Autodesk Inventor part; units mm, degrees
ref_plane "YZ Plane" through (0, 0, 0) normal (1, 0, 0) x (0, 1, 0)
ref_plane "XZ Plane" through (0, 0, 0) normal (0, 1, 0) x (-1, 0, 0)
ref_plane "XY Plane" through (0, 0, 0) normal (0, 0, 1) x (1, 0, 0)
sketch "スケッチ1" plane through (0, 0, 0) normal (0, 0, 1) x (1, 0, 0)
  line L0 (0, 2.3094) -> (2, 1.1547)
  line L1 (2, 1.1547) -> (2, -1.1547)
  line L2 (2, -1.1547) -> (0, -2.3094)
  line L3 (0, -2.3094) -> (-2, -1.1547)
  line L4 (-2, -1.1547) -> (-2, 1.1547)
  line L5 (-2, 1.1547) -> (0, 2.3094)
  point P0 (0, 0)
  point P1 (0, 0)
  dimension "d0" = 4
extrude "押し出し1" add sketch "スケッチ1" along normal blind 6
sketch "スケッチ2" plane through (0, 0, 6) normal (0, 0, 1) x (1, 0, 0)
  circle A0 centre (0, 0) radius 1
  dimension "d3" = 2
extrude "押し出し2" add sketch "スケッチ2" along normal blind 5
thread "ねじ1"
sketch "スケッチ3" plane through (0, 0, 0) normal (0, 0, -1) x (-1, 0, 0)
  point P0 (0, 0)
hole "穴1" at (0, 0, 0) direction (0, 0, 1) diameter 1.567 depth 4 tip angle 118
properties part number "ジュラコンスペーサー（六角）_BS-2006E" material "アセタール樹脂、白"
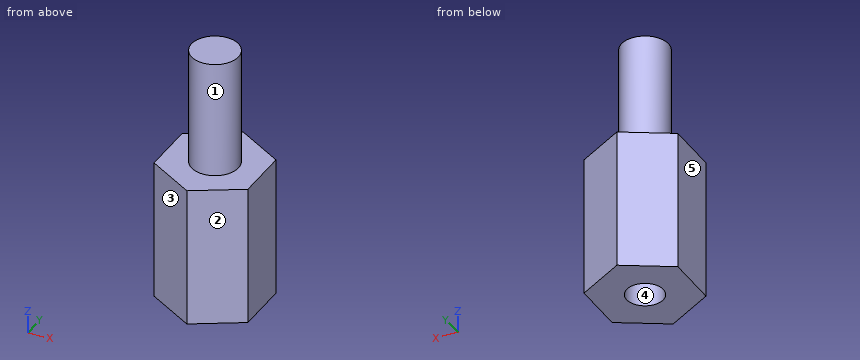
Read the model definition and answer for the solid it produces. Units are mm, in the model's axes. Face numbers are marked on the shaded views. A direction names the side the tool comes from. Round coordinates to 2 decimals unless told otherwise and drop trailing zeros. Order: outer loops, then holes, each group sorted by start corner. A loop starts at its lowest first (then second) coordinate and runs counter-clockwise, first axis right, second up. Notation, with made-up numbers: (87, 26) - (122, 26) arc R16 ccw to (122, 43) - close; hole circle Ø7 at (48, 69). An arc over 180 degrees is marked (long way). Use one line per item in the form item = value. Start each with the question number.
(1) For the marked faces 1 and 2, determine the directions among +Z, -Z, +X, -X, +Y, -Y from which every point of the face is accessible in a straight line to the end or side of a thin tool.
(2) Find the intervals of material crossed by line 1 along X through (y, z) = (0, 2.4); line 2 along Z through (x, y) = (1.75, -0.7); line 3 along Z through (x, y) = (0.4, -0.3), in increasing order. Write a range as from..to.
(3) Determine the mould class of the marked faces 3, 4 and 5 for opening direction Y: +Y half, -Y half, draft (parallel to the pull), parting line (faces both ways), or undercut.
(4) Flat-ended cylindrical pins translate along their axes: pin 1 Ø1 at (y, z) = (0.5, 7) entering from -X; pin 2 Ø1.5 at (x, z) = (-1, 3.5) entering from -Y. Find the tip coordinate at first contact, or state that the pin passes through.
(5) The part is cut by section C-C (y = -1.4). Give the vertices of the cut face in (x, z), then the cut area to 3 significant figures.
(6) The part is cut by section A-A (x = 1.6). Give the vertices of the cut face in (y, z).
(7) The part is cut by section B-B (z = 6.75). Give the vertices of the cut face in (x, y).
Checked values:
q1.face_1 = +Z
q1.face_2 = +Z, -Z, +X, -Y
q2.line_1 = -2..-0.78, 0.78..2
q2.line_2 = 0..6
q2.line_3 = 4.17..11
q3.face_3 = -Y half
q3.face_4 = undercut
q3.face_5 = draft
q4.pin_1 = -1
q4.pin_2 = -2.17
q5.outline = (-1.58, 0) - (1.58, 0) - (1.58, 6) - (-1.58, 6) - close
q5.area = 18.9 mm^2
q6.outline = (-1.39, 0) - (1.39, 0) - (1.39, 6) - (-1.39, 6) - close
q7.outline = circle Ø2 at (0, 0)
